CAD build for the part. Positions are in the model's coordinates, mm. Round coordinates to 2 decimals unless told otherwise and drop trailing zeros. Loops run counter-clockwise (first coordinate to the right, second up) from the corner with the lowest first, then second, coordinate; pieces in that order, holes last. Notation, with made-up numbers: M 38,34.25 L 52,34.25 A26 ccw 52,70.25 Z; hole C 31.25,-9.75 d4. An arc over 180 degrees is marked long. Use one line per item in the form item = value.
Autodesk Inventor part; units mm, degrees
ref_plane "YZ Plane" through (0, 0, 0) normal (1, 0, 0) x (0, 1, 0)
ref_plane "XZ Plane" through (0, 0, 0) normal (0, 1, 0) x (-1, 0, 0)
ref_plane "XY Plane" through (0, 0, 0) normal (0, 0, 1) x (1, 0, 0)
sketch "Sketch1" plane through (0, 0, 0) normal (0, 1, 0) x (-1, 0, 0)
  line L0 (-9.3478, 139.075) -> (-9.3478, 139.4112)
  line L1 (2.5473, 133.0612) -> (47.8022, 133.0612)
  line L2 (47.8022, 133.0612) -> (47.8022, 139.4112)
  line L3 (47.8022, 139.4112) -> (3.1135, 139.4112)
  line L4 (-2.9978, 139.4112) -> (-2.9978, 139.075)
  line L5 (-13.4187, 133.0612) -> (-60.1478, 133.0612)
  line L6 (-60.1478, 133.0612) -> (-60.1478, 139.075)
  line L7 (-60.1478, 139.075) -> (-14.0737, 139.075)
  line L8 (-9.3478, 189.875) -> (-2.9978, 189.875)
  line L9 (-9.3478, 128.9903) -> (-9.3478, 82.2612)
  line L10 (-9.3478, 82.2612) -> (-2.9978, 82.2612)
  line L11 (-2.9978, 82.2612) -> (-2.9978, 128.4241)
  line L12 (-14.9607, 189.7858) -> (4.0893, 189.7858)
  line L13 (4.0893, 189.7858) -> (4.0893, 208.8358)
  line L14 (4.0893, 208.8358) -> (-14.9607, 208.8358)
  line L15 (-14.9607, 208.8358) -> (-14.9607, 189.7858)
  line L16 (-60.1478, 146.4982) -> (-79.1978, 146.4982)
  line L17 (-79.1978, 146.4982) -> (-79.1978, 127.4482)
  line L18 (-79.1978, 127.4482) -> (-60.1478, 127.4482)
  line L19 (-60.1478, 127.4482) -> (-60.1478, 146.4982)
  line L20 (4.0893, 82.3504) -> (-14.9607, 82.3504)
  line L21 (-14.9607, 82.3504) -> (-14.9607, 63.3004)
  line L22 (-14.9607, 63.3004) -> (4.0893, 63.3004)
  line L23 (4.0893, 63.3004) -> (4.0893, 82.3504)
  line L24 (47.8022, 146.4982) -> (66.8522, 146.4982)
  line L25 (66.8522, 146.4982) -> (66.8522, 127.4482)
  line L26 (66.8522, 127.4482) -> (47.8022, 127.4482)
  line L27 (47.8022, 127.4482) -> (47.8022, 146.4982)
  circle A0 centre (-5.4357, 136.9732) radius 8.89
  line L28 (-9.3478, 139.075) -> (-9.3478, 139.4112)
  line L29 (-9.3478, 144.9562) -> (-9.3478, 189.875)
  line L30 (-2.9978, 189.875) -> (-2.9978, 145.5224)
  line L31 (-2.9978, 139.4112) -> (-2.9978, 139.075)
extrude "Extrusion1" add sketch "Sketch1" along normal blind 6.35
sketch "Sketch2" plane through (0, 6.35, 0) normal (0, 1, 0) x (1, 0, 0)
  line L0 (-47.8022, -139.4112) -> (-3.1135, -139.4112)
  circle A0 centre (5.4822, -136.8972) radius 8.9557
  circle A1 centre (5.4822, -136.8972) radius 10.5259
  point P0 (0, 0)
extrude "Extrusion2" add sketch "Sketch2" along normal blind 2.794
sketch "Sketch3" plane through (0, 6.35, 0) normal (0, 1, 0) x (1, 0, 0)
  point P0 (0, 0)
hole "Hole1" at (1.0354, 0, 140.8984) direction (0, 1, 0) diameter 3.81 end through all counterbore diameter 4.826 counterbore depth 3.81
hole "Hole2" at (9.6697, 0, 132.9413) direction (0, 1, 0) diameter 3.81 end through all counterbore diameter 4.826 counterbore depth 3.81
hole "Hole3" at (9.5106, 0, 141.2132) direction (0, 1, 0) diameter 3.81 end through all counterbore diameter 4.826 counterbore depth 3.81
hole "Hole4" at (1.3978, 0, 132.6231) direction (0, 1, 0) diameter 3.81 end through all counterbore diameter 4.826 counterbore depth 3.81
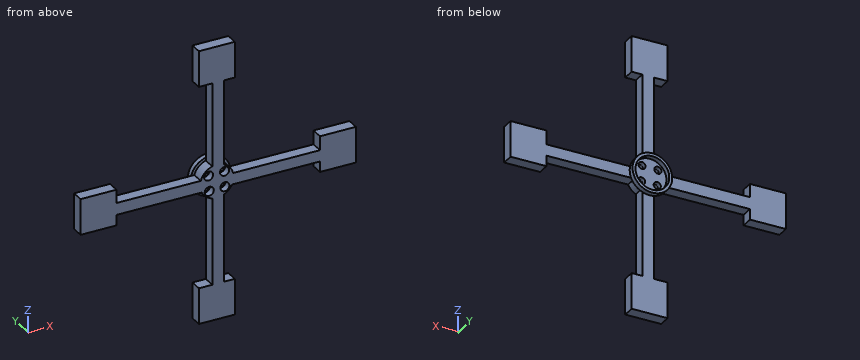
1. Cut at A-A on x = 24. Write the cut outline in (y, z) (3 decimals), and give its area (3 significant figures).
Completed:
outline = M 0,133.061 L 6.35,133.061 L 6.35,139.075 L 0,139.075 Z
area = 38.2 mm2
2. Cut at C-C on y = 1.5. State how many separate pieces and enclosed holes the cut face has, and give its area (3 significant figures).
Completed:
separate_pieces = 1
enclosed_holes = 4
area = 2,760 mm2
3. Cut at B-B on z = 164. Write the cut outline in (x, y), and give its area (3 significant figures).
Completed:
outline = M 3,0 L 9.35,0 L 9.35,6.35 L 3,6.35 Z
area = 40.3 mm2
4. Probe line 1 along X through (y, z) = (2, 169); line 2 along X through (y, z) = (5.5, 130.5); line 3 along Z through (x, y) = (70, 5). List the from-to ranges inside material, lowest first. Write a range as from..to.
Completed:
line_1 = 3..9.35
line_2 = -66.85..-47.8, -0.66..11.53, 60.15..79.2
line_3 = 127.45..146.5
5. Drop flat-ended pins along their axis: P1, Ø1.9, axis at x = -25.5, y = 4, coming from the +Z side; P2, Ø5, axis at y = 2, z = 96, coming from the +X side; P3, Ø3, axis at y = 4, z = 148.5, coming from the -X side. Give the stop position or say it passes through.
Completed:
P1 = 139.41
P2 = 9.35
P3 = 3
